Build history of the part. All positions in model axes, mm. A direction names the side the tool comes from. Give positions to 0.01 mm unless a question says otherwise; leave off trailing zeros. Order: outer loops, then holes, each group sorted by start corner. A loop starts at its lowest first (then second) coordinate and runs counter-clockwise, first axis right, second up. Notation, with made-up numbers: (61.5, -5) -> (107.5, -5) arc R13 cw to (107.5, 0) -> close; hole circle Ø6 at (48.5, 60.25). An arc over 180 degrees is marked (long way). Use a Markdown table: item, result. Add a question column.
```python
from build123d import *

# Parameters (mm, degrees)
F0_W           = 70
F0_H           = 114
F0_R           = 2.5
F0_W_2         = 11
F0_H_2         = 25
F1_DEPTH       = 5
F2_T           = -2.5
F4_D           = 5
F4_CSINK_D     = 10
F4_CSINK_ANGLE = 90
F5_R           = 4.99999


# Not quite as in the source:
# - a fillet or chamfer is up to 0.001 mm smaller than in the source, because OpenCascade refuses the exact size


with BuildPart() as f1:
    # F0 (on Front) → F1 (new body)
    with BuildSketch(Plane.XZ):
        Rectangle(F0_W, F0_H)
        with Locations((0, -30)):
            Circle(F0_R, mode=Mode.SUBTRACT)
        Rectangle(F0_W_2, F0_H_2, mode=Mode.SUBTRACT)
        with Locations((0, 30)):
            Circle(F0_R, mode=Mode.SUBTRACT)
    extrude(amount=F1_DEPTH)

    # F2
    f2_openings = [f1.faces().sort_by_distance(p)[0] for p in [
        (0, 0, -55.662241),
    ]]
    offset(amount=F2_T, openings=f2_openings, kind=Kind.INTERSECTION)

    # F4 (through all)
    with Locations(Plane.XZ.offset(5)):
        with Locations((0, 30), (0, -30)):
            CounterSinkHole(F4_D / 2, F4_CSINK_D / 2, counter_sink_angle=F4_CSINK_ANGLE)

    # F5 (radius 5 in the source; OpenCascade refuses exactly that, so slightly less here)
    f5_edges = [f1.edges().sort_by_distance(p)[0] for p in [
        (-35, -5, 0),
        (0, -5, 57),
        (35, -5, 0),
        (0, -5, -57),
    ]]
    fillet(f5_edges, radius=F5_R)


solid = f1.part
```
(1) Tool access for faces 1 (the face through (-5.5, -2, 0)), 2 (the face through (0.57, -2.62, 27.44)), 3 (the face through (0, -1, 54.5)): list every direction of +Z, -Z, +X, -X, +Y, -Y with a clear straight run to the whole face (end or side of a thin tool).
(2) Pin check, flat tips, straight feed: pin 1 Ø2 at (x, y) = (2, -1.5) entering from -Z; pin 2 Ø0.8 at (y, z) = (-1.5, 6.5) entering from -X; pin 3 Ø0.8 at (y, z) = (-1, -2.5) entering from +X. Stop position of each tip, or through.
(3) Mould opens along Z. For faces 4 (the face through (0, -4, -55)), 5 (the face through (2.31, -1.23, -30.96)), 6 (the face through (33, -4, 1)) say: released by +Z, released by -Z, zero draft, split by the parting line, or undercut.
(4) Band-saw the part on D-D on x = 0. State how many separate pieces and enclosed holes the cut face has, plus the area to 3 significant figures.
(5) Wall check: probe 1 along Z at (x, y) = (-24, -0.5); probe 2 along X at (y, z) = (-0.65, 0); probe 3 along X at (y, z) = (-2.05, 33.5). Give the ranges that are in metal, low to high.
(6) Band-saw the part on A-A on y = -1.4. Give the cut face in (x, z).
Response:
| question | item | result |
|---|---|---|
| 1 | face 1 | +Y, -Y |
| 1 | face 2 | -Y |
| 1 | face 3 | +Y |
| 2 | pin 1 | stops at z = -56.97 |
| 2 | pin 2 | stops at x = -34.88 |
| 2 | pin 3 | stops at x = 34.96 |
| 3 | face 4 | released by -Z |
| 3 | face 5 | undercut |
| 3 | face 6 | zero draft |
| 4 | separate pieces | 4 |
| 4 | enclosed holes | 0 |
| 4 | area | 224 mm² |
| 5 | probe 1 | z = -56.97 to -54.5, 54.5 to 56.97 |
| 5 | probe 2 | x = -34.96 to -32.5, -8 to -5.5, 5.5 to 8, 32.5 to 34.96 |
| 5 | probe 3 | x = -34.56 to -32.5, -3.57 to 3.57, 32.5 to 34.56 |
| 6 | outline | (-34.8, -56.8) -> (34.8, -56.8) -> (34.8, 56.8) -> (-34.8, 56.8) -> close; (-8, -15) -> (8, -15) -> (8, 15) -> (-8, 15) -> close; circle Ø10 at (0, -30); circle Ø10 at (0, 30); hole (-32.5, -54.5) -> (32.5, -54.5) -> (32.5, 54.5) -> (-32.5, 54.5) -> close; hole (-5.5, -12.5) -> (5.5, -12.5) -> (5.5, 12.5) -> (-5.5, 12.5) -> close; hole circle Ø5 at (0, -30); hole circle Ø5 at (0, 30) |
